```python
from build123d import *

# Parameters (mm, degrees)
F0_R     = 2.1
F1_DEPTH = 12
F2_R     = 2.1
F3_DEPTH = 15.001
F4_SIZE  = 1


with BuildPart() as f1:
    # F0 (on Top) → F1 (new body)
    with BuildSketch(Plane.XY):
        with BuildLine():
            Line((-8.417424, -9), (8.417424, -9))
            ThreePointArc((8.417424, -9), (9.512869, -8.67332), (10.250455, -7.8))
            ThreePointArc((10.250455, -7.8), (11.356832, -6.49002), (13, -6))
            Line((13, -6), (30, -6))
            ThreePointArc((30, -6), (36, 0), (30, 6))
            Line((30, 6), (-30, 6))
            ThreePointArc((-30, 6), (-36, 0), (-30, -6))
            Line((-30, -6), (-13, -6))
            ThreePointArc((-13, -6), (-11.356832, -6.49002), (-10.250455, -7.8))
            ThreePointArc((-10.250455, -7.8), (-9.512869, -8.67332), (-8.417424, -9))
        make_face()
        with Locations((-30, 0)):
            Circle(F0_R, mode=Mode.SUBTRACT)
        with Locations((30, 0)):
            Circle(F0_R, mode=Mode.SUBTRACT)
    extrude(amount=F1_DEPTH)

    # F2 (on face) → F3 (cut, through all)
    with BuildSketch(Plane(origin=(0, 6, 0), x_dir=(-1, 0, 0), z_dir=(0, 1, 0))):
        with Locations((0, 6)):
            Circle(F2_R)
    extrude(amount=-F3_DEPTH, mode=Mode.SUBTRACT)

    # F4
    f4_edges = [f1.edges().sort_by_distance(p)[0] for p in [
        (0, -9, 12),
        (0, 6, 0),
    ]]
    chamfer(f4_edges, length=F4_SIZE)


solid = f1.part
```
Could you check a few things on this model? Use its own coordinates, in mm. A direction names the side the tool comes from. Round coordinates to 2 decimals unless told otherwise and drop trailing zeros. Loops run counter-clockwise (first coordinate to the right, second up) from the corner with the lowest first, then second, coordinate; pieces in that order, holes last.
Q1. I want a section at A-A (z = 6). Write out the boundary of the cut face in (x, y).
Q2. Thinking about a two-plate mould opening in Z: for faces 3 (the cylindrical face through (0.273, -1.395, 8.082)), 4 (the flat face through (-22, -6, 6)), 5 (the flat face through (0, 0, 12)), which applies, pulls with the +Z half, pulls with the -Z half, needs draft (parallel to the pull), parting line crosses it, or undercut?
Q3. Please list where these lines run through material, in increasing order: L1, parallel to Y at x = -30, z = 8.25; L2, parallel to X at y = 1, z = 7.75; L3, parallel to Z at x = 0, y = -3.
Q4. I want a section at C-C (y = 0). Write out the boundary of the cut face in (x, z).
Q5. I want a section at B-B (x = 0). Write out the boundary of the cut face in (y, z), and give its area (3 significant figures).
Q6. For P1, Ø4, axis at y = -2.5, z = 6.5, coming from the +X side; P2, Ø5.5, axis at x = 30, y = 0, coming from the +Z side, each with a flat end and sliding along its axis, tell me the tip position at first contact or that it passes through.
Q7. I want a section at D-D (z = 9.25). Write out the boundary of the cut face in (x, y).
Q8. On a 3-axis mill with a long thin cutter (end or side, diameter ignored), from which of +Z, -Z, +X, -X, +Y, -Y can I reach the whole of each face in a straight line? I mean faces 1 (the cylindrical face through (-36, 0, 6)), 2 (the flat face through (21, -6, 6)). Say none if no direction works.
Answer below:
1. outline: (-30, -6) - (-13, -6) arc R3 cw to (-10.25, -7.8) arc R2 ccw to (-8.42, -9) - (-2.1, -9) - (-2.1, 6) - (-30, 6) arc R6 ccw to start; (2.1, -9) - (8.42, -9) arc R2 ccw to (10.25, -7.8) arc R3 cw to (13, -6) - (30, -6) arc R6 ccw to (30, 6) - (2.1, 6) - close; hole circle Ø4.2 at (-30, 0); hole circle Ø4.2 at (30, 0)
2. face 3: undercut
2. face 4: needs draft
2. face 5: pulls with the +Z half
3. L1: y = -6 to -2.1, 2.1 to 6
3. L2: x = -35.92 to -31.85, -28.15 to -1.16, 1.16 to 28.15, 31.85 to 35.92
3. L3: z = 0 to 3.9, 8.1 to 12
4. outline: (-36, 1) - (-35, 0) - (-32.1, 0) - (-32.1, 12) - (-35, 12) - (-36, 11) - close; (-27.9, 0) - (27.9, 0) - (27.9, 12) - (-27.9, 12) - close; (32.1, 0) - (35, 0) - (36, 1) - (36, 11) - (35, 12) - (32.1, 12) - close; hole circle Ø4.2 at (0, 6)
5. outline: (-9, 1) - (-8, 0) - (5, 0) - (6, 1) - (6, 3.9) - (-9, 3.9) - close; (-9, 8.1) - (6, 8.1) - (6, 11) - (5, 12) - (-8, 12) - (-9, 11) - close
5. area: 115 mm2
6. P1: stops at x = 35.98
6. P2: stops at z = 12
7. outline: (-30, -6) - (-13, -6) arc R3 cw to (-10.25, -7.8) arc R2 ccw to (-8.42, -9) - (8.42, -9) arc R2 ccw to (10.25, -7.8) arc R3 cw to (13, -6) - (30, -6) arc R6 ccw to (30, 6) - (-30, 6) arc R6 ccw to start; hole circle Ø4.2 at (-30, 0); hole circle Ø4.2 at (30, 0)
8. face 1: +Z, -Z, -X
8. face 2: +Z, -Z, +X, -Y
